CAD build for the part. Positions are in the model's coordinates, mm. Face numbers are marked on the shaded views. A direction names the side the tool comes from. Coordinates: 2 decimals unless noted, no trailing zeros. Order: outer loops, then holes, each group sorted by start corner. A loop starts at its lowest first (then second) coordinate and runs counter-clockwise, first axis right, second up.
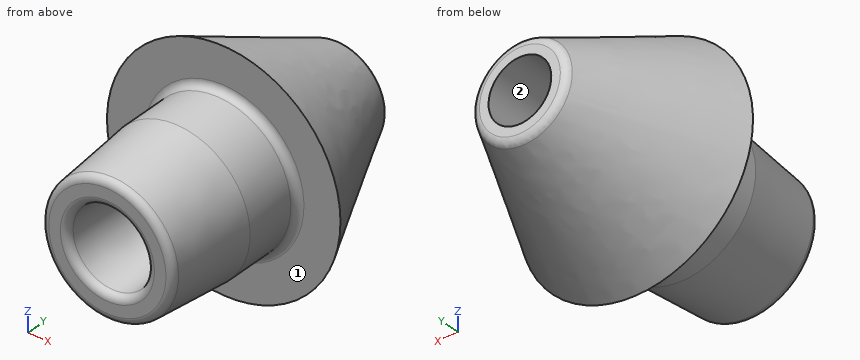
from build123d import *

# Parameters (mm, degrees)
SKETCH1_R           = 2.5
BOSS_EXTRUDE1_DEPTH = 5
SKETCH4_R           = 1.075
CUT_EXTRUDE1_DEPTH  = 12.489125363
CHAMFER1_SIZE       = 0.3
CHAMFER1_SIZE2      = 5.724341006
CHAMFER2_SIZE       = 3
CHAMFER2_SIZE2      = 0.262465991
FILLET1_R           = 0.3
FILLET2_R           = 0.25
FILLET4_R           = 0.25


with BuildPart() as part:
    # Sketch1 → Boss-Extrude1 (new body)
    with BuildSketch(Plane(origin=(0, 0, 0), x_dir=(1, 0, 0), z_dir=(0, 1, 0))):
        with Locations(Location((0, 0, 0), (0, 0, 270))):
            Circle(SKETCH1_R)
    extrude(amount=BOSS_EXTRUDE1_DEPTH)

    # Loft1: read off the stored shape, not the designer's step
    # Loft1: loft between two sections, ruled curve by curve
    loft1_from = [
        Edge.make_bspline([(-1.392393657, 10, -0.736114736), (0.079835815, 10, -3.52090205), (2.864623129, 10, -2.048672577), (1.392393657, 10, 0.736114736), (-0.079835815, 10, 3.52090205), (-2.864623129, 10, 2.048672577), (-1.392393657, 10, -0.736114736)], [0, 0, 0, 0, 0.5, 0.5, 0.5, 1, 1, 1, 1], 3, [1, 0.333333333, 0.333333333, 1, 0.333333333, 0.333333333, 1]),
    ]
    loft1_to = [
        Edge.make_bspline([(-3.843967333, 5, -1.106306985), (-1.631353363, 5, -8.79424165), (6.056581302, 5, -6.581627681), (3.843967333, 5, 1.106306985), (1.631353363, 5, 8.79424165), (-6.056581302, 5, 6.581627681), (-3.843967333, 5, -1.106306985)], [0, 0, 0, 0, 0.5, 0.5, 0.5, 1, 1, 1, 1], 3, [1, 0.333333333, 0.333333333, 1, 0.333333333, 0.333333333, 1]),
    ]
    loft1 = Solid(Shell([*[Face.make_surface_from_curves(loft1_from[k], loft1_to[k]) for k in range(1)], Face(Wire(loft1_from)), Face(Wire(loft1_to))]))
    add(loft1)

    # Sketch4 → Cut-Extrude1 (cut, through all)
    with BuildSketch(Plane(origin=(0, 10, 0), x_dir=(1, 0, 0), z_dir=(0, 1, 0))):
        with Locations(Location((0, 0, 0), (0, 0, 270))):
            Circle(SKETCH4_R)
    extrude(amount=-CUT_EXTRUDE1_DEPTH, mode=Mode.SUBTRACT)

    # Chamfer1
    chamfer1_edges = [part.edges().sort_by_distance(p)[0] for p in [
        (0, 0, -1.075),
    ]]
    chamfer1_side = [part.faces().sort_by_distance(p)[0] for p in [
        (0, 0, -2.429289322),
    ]]
    chamfer(chamfer1_edges, length=CHAMFER1_SIZE, length2=CHAMFER1_SIZE2, reference=chamfer1_side[0])

    # Chamfer2
    chamfer2_edges = [part.edges().sort_by_distance(p)[0] for p in [
        (0, 0, -2.5),
    ]]
    chamfer2_side = [part.faces().sort_by_distance(p)[0] for p in [
        (0, 2.5, -2.5),
    ]]
    chamfer(chamfer2_edges, length=CHAMFER2_SIZE, length2=CHAMFER2_SIZE2, reference=chamfer2_side[0])

    # Fillet1
    fillet1_edges = [part.edges().sort_by_distance(p)[0] for p in [
        (1.392393657, 10, 0.736114736),
    ]]
    fillet(fillet1_edges, radius=FILLET1_R)

    # Fillet2
    fillet2_edges = [part.edges().sort_by_distance(p)[0] for p in [
        (0, 5, -2.5),
    ]]
    fillet(fillet2_edges, radius=FILLET2_R)

    # Fillet4
    fillet4_edges = [part.edges().sort_by_distance(p)[0] for p in [
        (0, 0, -1.375),
        (0, 0, -2.237534009),
    ]]
    fillet(fillet4_edges, radius=FILLET4_R)


solid = part.part
1) Drill centre lines: probe 1 along Z at (x, y) = (0.75, 0.75); probe 2 along X at (y, z) = (8.6, 0) (3 decimals); probe 3 along Z at (x, y) = (-0.5, 1.25). Where is each one in solid material? Low to high.
2) Which spindle directions (+Z, -Z, +X, -X, +Y, -Y) get a long thin tool onto all of the face, cutting with end or side? Do the marked faces 1 and 2. Say none if no direction does.
3) Slice it at B-B (y = 3.5). List the corners of the cut face in (x, z), plus the area to 3 significant figures.
4) Slice it at A-A (y = 2). List the corners of the cut face in (x, z).
5) Pin check, flat tips, straight feed: P1, Ø2, axis at x = -2.5, y = 1.5, coming from the -Z side; P2, Ø4, axis at x = -2, y = 4, coming from the -Z side. Stop position of each tip, or through.
Worked out:
1. probe 1: z = -2.18 to -1.11, 1.11 to 2.18
1. probe 2: x = -2.242 to -1.075, 1.075 to 2.242
1. probe 3: z = -2.29 to -1.21, 1.21 to 2.29
2. face 1: -Y
2. face 2: +Y, -Y
3. outline: circle Ø5 at (0, 0); hole circle Ø2.38 at (0, 0)
3. area: 15.2 mm2
4. outline: circle Ø4.83 at (0, 0); hole circle Ø2.54 at (0, 0)
5. P1: stops at z = -1.84
5. P2: stops at z = -3.99
